Read the model definition and answer for the solid it produces. Units are mm, in the model's axes. A direction names the side the tool comes from. Round coordinates to 2 decimals unless told otherwise and drop trailing zeros. Order: outer loops, then holes, each group sorted by start corner. A loop starts at its lowest first (then second) coordinate and runs counter-clockwise, first axis right, second up. Notation, with made-up numbers: (-38, -1) -> (-3, -1) arc R19 ccw to (-3, 25) -> close; hole circle Ø6 at (76.25, 60). An arc over 180 degrees is marked (long way). One line per item, written item: value. Start each with the question number.
1. Consider line 1 (X direction, y = 3.75, z = 7); line 2 (X direction, y = 0, z = 50); line 3 (Z direction, x = 9.25, y = -0.25). Determine where each line is inside the solid, lowest interval first.
2. Section C-C (y = -6.5) is taken. Give the vertices of the cut face in (x, z), then the cut area to 3 significant figures.
3. For faces 1 (the face through (0, 0, 47)), 2 (the face through (-11.5, 0, 95)), 3 (the face through (-8, 0, 3)), 4 (the face through (0, 8, 97)), 5 (the face through (2.5, 7, 5)), determine the directions among +Z, -Z, +X, -X, +Y, -Y from which every point of the face is accessible in a straight line to the end or side of a thin tool.
4. Section D-D (x = 0) is taken. Give the vertices of the cut face in (y, z), then the cut area to 3 significant figures.
5. The mould has two halves that part along Z. Classify faces 6 (the face through (2.5, -5, 95)), 7 (the face through (0, 8, 95)), 8 (the face through (-3, 0, 0)): released by +Z, released by -Z, zero draft, split by the parting line, or undercut.
6. Section B-B (z = 50) is taken. Give the vertices of the cut face in (x, y).
7. Section A-A (y = 0.5) is taken. Give the vertices of the cut face in (x, z), then the cut area to 3 significant figures.
from build123d import *

# Parameters (mm, degrees)
ESQUISSE1_W             = 25
ESQUISSE1_H             = 25
BOSS_EXTRU_1_DEPTH      = 100
ENL_V_MAT_EXTRU_2_DEPTH = 10
ESQUISSE9_R             = 3
ENL_V_MAT_EXTRU_4_DEPTH = 54
ENL_V_MAT_EXTRU_5_DEPTH = 10
ESQUISSE10_W            = 5
ESQUISSE10_H            = 2
ENL_V_MAT_EXTRU_6_DEPTH = 13
ESQUISSE11_W            = 2
ESQUISSE11_H            = 5
ENL_V_MAT_EXTRU_7_DEPTH = 13


with BuildPart() as part:
    # Esquisse1 → Boss.-Extru.1 (new body)
    with BuildSketch(Plane.XY):
        Rectangle(ESQUISSE1_W, ESQUISSE1_H)
    extrude(amount=BOSS_EXTRU_1_DEPTH)

    # Esquisse3 → Enlèv. mat.-Extru.2 (cut)
    with BuildSketch(Plane.XY.offset(100)):
        Polygon((-11.5, 2.5), (11.5, 2.5), (11.5, -2.5), (2.5, -2.5), (2.5, -7.5), (-2.5, -7.5), (-2.5, -2.5), (-11.5, -2.5), align=None)
    extrude(amount=-ENL_V_MAT_EXTRU_2_DEPTH, mode=Mode.SUBTRACT)

    # Esquisse9 → Enlèv. mat.-Extru.4 (cut)
    with BuildSketch(Plane(origin=(0, 12.5, 0), x_dir=(1, 0, 0), z_dir=(0, 1, 0))):
        with Locations(Location((0, -50, 0), (0, 0, 270))):
            Circle(ESQUISSE9_R)
    extrude(amount=-ENL_V_MAT_EXTRU_4_DEPTH, mode=Mode.SUBTRACT)

    # Esquisse4 → Enlèv. mat.-Extru.5 (cut)
    with BuildSketch(Plane.XY):
        Polygon((2.5, 11.5), (-2.5, 11.5), (-2.5, -11.5), (2.5, -11.5), (2.5, -2.5), (7.5, -2.5), (7.5, 2.5), (2.5, 2.5), align=None)
    extrude(amount=ENL_V_MAT_EXTRU_5_DEPTH, mode=Mode.SUBTRACT)

    # Esquisse10 → Enlèv. mat.-Extru.6 (cut)
    with BuildSketch(Plane(origin=(0, 12.5, 0), x_dir=(1, 0, 0), z_dir=(0, 1, 0))):
        with Locations((0, -96)):
            Rectangle(ESQUISSE10_W, ESQUISSE10_H)
    extrude(amount=-ENL_V_MAT_EXTRU_6_DEPTH, mode=Mode.SUBTRACT)

    # Esquisse11 → Enlèv. mat.-Extru.7 (cut)
    with BuildSketch(Plane.ZY.offset(12.5)):
        with Locations((4, 0)):
            Rectangle(ESQUISSE11_W, ESQUISSE11_H)
    extrude(amount=-ENL_V_MAT_EXTRU_7_DEPTH, mode=Mode.SUBTRACT)


solid = part.part
Answer:
1. line 1: -12.5 to -2.5, 2.5 to 12.5
1. line 2: -12.5 to -3, 3 to 12.5
1. line 3: 0 to 90
2. outline: (-12.5, 0) -> (-2.5, 0) -> (-2.5, 10) -> (2.5, 10) -> (2.5, 0) -> (12.5, 0) -> (12.5, 100) -> (2.5, 100) -> (2.5, 90) -> (-2.5, 90) -> (-2.5, 100) -> (-12.5, 100) -> close; hole circle Ø6 at (0, 50)
2. area: 2,370 mm^2
3. face 1: +Y, -Y
3. face 2: +Z
3. face 3: -X
3. face 4: +Y
3. face 5: -Z
4. outline: (-12.5, 0) -> (-11.5, 0) -> (-11.5, 10) -> (11.5, 10) -> (11.5, 0) -> (12.5, 0) -> (12.5, 47) -> (-12.5, 47) -> close; (-12.5, 53) -> (12.5, 53) -> (12.5, 95) -> (2.5, 95) -> (2.5, 90) -> (-7.5, 90) -> (-7.5, 100) -> (-12.5, 100) -> close; (2.5, 97) -> (12.5, 97) -> (12.5, 100) -> (2.5, 100) -> close
4. area: 2,000 mm^2
5. face 6: zero draft
5. face 7: undercut
5. face 8: released by -Z
6. outline: (-12.5, -12.5) -> (-3, -12.5) -> (-3, 12.5) -> (-12.5, 12.5) -> close; (3, -12.5) -> (12.5, -12.5) -> (12.5, 12.5) -> (3, 12.5) -> close
7. outline: (-12.5, 0) -> (-2.5, 0) -> (-2.5, 3) -> (-12.5, 3) -> close; (-12.5, 5) -> (-2.5, 5) -> (-2.5, 10) -> (7.5, 10) -> (7.5, 0) -> (12.5, 0) -> (12.5, 100) -> (11.5, 100) -> (11.5, 90) -> (-11.5, 90) -> (-11.5, 100) -> (-12.5, 100) -> close; hole circle Ø6 at (0, 50)
7. area: 2,120 mm^2
